from build123d import *

# Parameters (mm, degrees)
BOSS_EXTRUDE1_DEPTH = 20
SKETCH2_R           = 2
SKETCH2_R_2         = 0.5
CUT_EXTRUDE1_DEPTH  = 299.872882678
CUT_EXTRUDE2_START  = -2
CUT_EXTRUDE2_DEPTH  = 239


with BuildPart() as part:
    # Sketch1 → Boss-Extrude1 (new, symmetric)
    with BuildSketch(Plane(origin=(0, 0, 0), x_dir=(1, 0, 0), z_dir=(0, 1, 0))):
        with BuildLine():
            Line((-117.5, -10), (-117.5, 10))
            Line((-117.5, 10), (-117.5, 47.5))
            ThreePointArc((-117.5, 47.5), (0, 165), (117.5, 47.5))
            Line((117.5, 47.5), (117.5, 10))
            Line((117.5, 10), (117.5, -10))
            Line((117.5, -10), (122.5, -10))
            Line((122.5, -10), (122.5, 47.5))
            ThreePointArc((122.5, 47.5), (0, 170), (-122.5, 47.5))
            Line((-122.5, 47.5), (-122.5, -10))
            Line((-122.5, -10), (-117.5, -10))
        make_face()
    extrude(amount=BOSS_EXTRUDE1_DEPTH, both=True)

    # Sketch2 → Cut-Extrude1 (cut, through all)
    with BuildSketch(Plane.ZY.offset(122.5)):
        Circle(SKETCH2_R)
        with Locations((4, 0)):
            Circle(SKETCH2_R_2)
        with Locations((6, 0)):
            Circle(SKETCH2_R_2)
        with Locations((-6, 0)):
            Circle(SKETCH2_R_2)
        with Locations((-4, 0)):
            Circle(SKETCH2_R_2)
        with Locations((0, 4.5)):
            Circle(SKETCH2_R_2)
        with Locations((0, 6.5)):
            Circle(SKETCH2_R_2)
        with Locations((0, 8.5)):
            Circle(SKETCH2_R_2)
        with Locations((0, 10.5)):
            Circle(SKETCH2_R_2)
        with Locations((0, 12.5)):
            Circle(SKETCH2_R_2)
        with Locations((0, -12.5)):
            Circle(SKETCH2_R_2)
        with Locations((0, -10.5)):
            Circle(SKETCH2_R_2)
        with Locations((0, -8.5)):
            Circle(SKETCH2_R_2)
        with Locations((0, -6.5)):
            Circle(SKETCH2_R_2)
        with Locations((0, -4.5)):
            Circle(SKETCH2_R_2)
    extrude(amount=-CUT_EXTRUDE1_DEPTH, mode=Mode.SUBTRACT)

    # Sketch3 → Cut-Extrude2 (cut)
    with BuildSketch(Plane(origin=(-117.5, 0, 0), x_dir=(0, 0, -1), z_dir=(1, 0, 0)).offset(CUT_EXTRUDE2_START)):
        Polygon((-8.25, 3), (-8.25, -3), (-3, -3), (-3, -15.25), (3, -15.25), (3, -3), (8.25, -3), (8.25, 3), (3, 3), (3, 15.25), (-3, 15.25), (-3, 3), align=None)
    extrude(amount=CUT_EXTRUDE2_DEPTH, mode=Mode.SUBTRACT)


solid = part.part
The model under review builds one solid part; all positions refer to its coordinate system, in mm. A direction names the side the tool comes from. Give positions to 0.01 mm unless a question says otherwise; leave off trailing zeros. Order: outer loops, then holes, each group sorted by start corner. A loop starts at its lowest first (then second) coordinate and runs counter-clockwise, first axis right, second up. Notation, with made-up numbers: M -22.5,-0.75 L 12.5,-0.75 A35 ccw 12.5,32.25 Z; hole C -1.5,-10 d11. An arc over 180 degrees is marked long. Use one line per item in the form item = value. Start each with the question number.
Item 1: We need section B-B on z = -137. Give the boundary of the cut face in (x, y), plus the area to 3 significant figures.
Item 2: Insertion check: pin 1 Ø3.5 at (y, z) = (0, 0) entering from -X; pin 2 Ø10 at (y, z) = (-16, -78.5) entering from +X; pin 3 Ø2 at (y, z) = (0, -122) entering from +X; pin 4 Ø3 at (y, z) = (13.5, -137.5) entering from -X. Each pin has a flat end and moves straight along its axis. Give the tip position at first contact, or say it passes through.
Item 3: To check wall thickness, follow line 1 along X through (y, z) = (-12, -28.5); line 2 along X through (y, z) = (14, -81); line 3 along Z through (x, y) = (-31.5, -2.5). State the ranges of each line that lie inside material, in increasing order. Write a range as from..to.
Item 4: The part is to be moulded in two halves that separate along Y. For faces 3 (the flat face through (-37, 20, -160)), 4 (the flat face through (119.5, -1, 2)), 5 (the flat face through (-119.5, -1, 2)), 6 (the flat face through (122.5, 0, -18)), say which applies: pulls with the +Y half, pulls with the -Y half, needs draft (parallel to the pull), parting line crosses it, or undercut.
Item 5: For faces 1 (the flat face through (-122.5, 0, -19)), 2 (the flat face through (117.5, 0, -19)), list the 3-axis set-ups (+Z, -Z, +X, -X, +Y, -Y) from which the entire face can be reached by the end or side of a thin tool; tool diameter is ignored.
Item 6: We need section A-A on z = -12. Give the boundary of the cut face in (x, y).
Item 7: We need section D-D on x = -102.5. Give the boundary of the cut face in (y, z), plus the area to 3 significant figures.
Item 8: We need section C-C on x = 100.5. Give the boundary of the cut face in (y, z).
Completed:
q1.outline = M -83.64,-20 L -76.13,-20 L -76.13,20 L -83.64,20 Z; M 76.13,-20 L 83.64,-20 L 83.64,20 L 76.13,20 Z
q1.area = 601 mm²
q2.pin_1 = through
q2.pin_2 = 119.71
q2.pin_3 = 98
q2.pin_4 = -84.7
q3.line_1 = -122.5..-117.5, 117.5..122.5
q3.line_2 = -117.83..-112.62, 112.62..117.83
q3.line_3 = -165.88..-160.7
q4.face_3 = pulls with the +Y half
q4.face_4 = undercut
q4.face_5 = undercut
q4.face_6 = needs draft
q5.face_1 = +Z, -Z, -X, +Y, -Y
q5.face_2 = +Z, +Y, -Y
q6.outline = M -122.5,-20 L -117.5,-20 L -117.5,20 L -122.5,20 Z; M 117.5,-20 L 122.5,-20 L 122.5,20 L 117.5,20 Z
q7.outline = M -20,-114.58 L 20,-114.58 L 20,-104.95 L -20,-104.95 Z
q7.area = 385 mm²
q8.outline = M -20,-117.54 L 20,-117.54 L 20,-108.38 L -20,-108.38 Z
